Geometry: final body of the model. Coordinates: model frame, mm. A direction names the side the tool comes from. Give positions to 0.01 mm unless a question says otherwise; leave off trailing zeros. Write each loop counter-clockwise with the first axis right and the second up, starting at its lowest first coordinate (ties: lowest second). Pieces come first, ordered by that corner, then holes. Notation, with made-up numbers: (7.25, 63) -> (42.25, 63) arc R11 cw to (42.25, 83) -> close; hole circle Ø7 at (-7, -22). An arc over 180 degrees is marked (long way). Answer in a Markdown table with one row per item. Add a question column.
Item 1: Access query for faces 1 (the cylindrical face through (-88.645, 29.462, -31.871)), 2 (the cylindrical face through (-45.58, 1.04, -25.25)), 3 (the cylindrical face through (-84.923, 14.183, -34.226)). Directions: +Z, -Z, +X, -X, +Y, -Y. A direction counts if a zero-diameter tool reaches every point of the face in a straight line with its end or side. Return the directions, or none.
Item 2: Section query D-D on z = -28. State how many separate pieces and enclosed holes the cut face has, plus the area to 3 significant figures.
Item 3: First-contact query: P1, Ø1.5, axis at x = -87.5, z = -22, coming from the +Y side (3 decimals); P2, Ø1, axis at x = -77, z = -31, coming from the -Y side. Flat tips, straight axial feed; report the tip coordinate or a pass-through.
Item 4: Section query C-C on y = 20. Output: boundary loops of the cut face in (x, z).
Item 5: Section query A-A on y = 15.5. Output: boundary loops of the cut face in (x, z).
Item 6: Material intervals for probe 1 along X at (y, z) = (10, -29.75); probe 2 along Y at (x, z) = (-79, -20.25) (3 decimals); probe 3 along X at (y, z) = (16, -30.5), sorted ascending. Write a range as from..to.
Item 7: Draft query along X for faces 4 (the flat face through (-74, 19.05, -26)), 5 (the cylindrical face through (-64.645, 29.462, -31.871)), 6 (the flat face through (-44, 0, -27)). Return one class per face: +X half, -X half, draft (parallel to the pull), parting line (faces both ways), or undercut.
```python
from build123d import *

# Parameters (mm, degrees)
SKETCH1_W           = 55.5625
SKETCH1_H           = 31.75
BOSS_EXTRUDE1_DEPTH = 28.575
SKETCH2_R           = 7.62
CUT_EXTRUDE1_DEPTH  = 13.335
CUT_EXTRUDE2_DEPTH  = 12.7
SKETCH4_R           = 1.8415
CUT_EXTRUDE3_DEPTH  = 25.4
CUT_EXTRUDE4_DEPTH  = 17.78
SKETCH6_W           = 55.5625
SKETCH6_H           = 28.575
CUT_EXTRUDE5_DEPTH  = 15.875
SKETCH7_R           = 2.778125
CUT_EXTRUDE7_DEPTH  = 7.9375
SKETCH8_R           = 2.35
BOSS_EXTRUDE2_DEPTH = 1.8
SKETCH9_R           = 3.25
SKETCH9_R_2         = 2.425
CUT_EXTRUDE8_DEPTH  = 2.1


with BuildPart() as part:
    # Sketch1 → Boss-Extrude1 (new body)
    with BuildSketch(Plane(origin=(0, 0, 0), x_dir=(1, 0, 0), z_dir=(0, 1, 0))):
        with Locations((-66.667749699, 35.16562105)):
            Rectangle(SKETCH1_W, SKETCH1_H)
    extrude(amount=BOSS_EXTRUDE1_DEPTH)

    # Sketch2 → Cut-Extrude1 (cut)
    with BuildSketch(Plane.XY.offset(-19.29062105)):
        with Locations((-54.761499699, 14.2875)):
            Circle(SKETCH2_R)
    extrude(amount=-CUT_EXTRUDE1_DEPTH, mode=Mode.SUBTRACT)

    # Sketch3 → Cut-Extrude2 (cut)
    with BuildSketch(Plane.XY.offset(-19.29062105)):
        with BuildLine():
            Line((-80.161499699, 19.05), (-67.461499699, 19.05))
            ThreePointArc((-67.461499699, 19.05), (-62.698999699, 14.2875), (-67.461499699, 9.525))
            Line((-67.461499699, 9.525), (-80.161499699, 9.525))
            ThreePointArc((-80.161499699, 9.525), (-84.923999699, 14.2875), (-80.161499699, 19.05))
        make_face()
    extrude(amount=-CUT_EXTRUDE2_DEPTH, mode=Mode.SUBTRACT)

    # Sketch4 → Cut-Extrude3 (cut)
    with BuildSketch(Plane.XY.offset(-31.99062105)):
        with Locations((-80.161499699, 14.2875)):
            Circle(SKETCH4_R)
        with Locations((-67.461499699, 14.2875)):
            Circle(SKETCH4_R)
    extrude(amount=-CUT_EXTRUDE3_DEPTH, mode=Mode.SUBTRACT)

    # Sketch5 → Cut-Extrude4 (cut)
    with BuildSketch(Plane(origin=(0, 0, -51.04062105), x_dir=(-1, 0, 0), z_dir=(0, 0, -1))):
        with BuildLine():
            Line((67.461499699, 9.525), (80.161499699, 9.525))
            ThreePointArc((80.161499699, 9.525), (84.923999699, 14.2875), (80.161499699, 19.05))
            Line((80.161499699, 19.05), (67.461499699, 19.05))
            ThreePointArc((67.461499699, 19.05), (62.698999699, 14.2875), (67.461499699, 9.525))
        make_face()
    extrude(amount=-CUT_EXTRUDE4_DEPTH, mode=Mode.SUBTRACT)

    # Sketch6 → Cut-Extrude5 (cut)
    with BuildSketch(Plane(origin=(0, 0, -51.04062105), x_dir=(-1, 0, 0), z_dir=(0, 0, -1))):
        with Locations((66.667749699, 14.2875)):
            Rectangle(SKETCH6_W, SKETCH6_H)
    extrude(amount=-CUT_EXTRUDE5_DEPTH, mode=Mode.SUBTRACT)

    # Sketch7 → Cut-Extrude7 (cut)
    with BuildSketch(Plane.XY.offset(-32.62562105)):
        with Locations((-54.761499699, 14.2875)):
            Circle(SKETCH7_R)
    extrude(amount=-CUT_EXTRUDE7_DEPTH, mode=Mode.SUBTRACT)

    # Sketch8 → Boss-Extrude2 (add)
    with BuildSketch(Plane(origin=(0, 28.575, 0), x_dir=(1, 0, 0), z_dir=(0, 1, 0))):
        with Locations((-42.886499699, 31.16562105)):
            Circle(SKETCH8_R)
        with Locations((-42.886499699, 23.16562105)):
            Circle(SKETCH8_R)
        with Locations((-50.886499699, 31.16562105)):
            Circle(SKETCH8_R)
        with Locations((-50.886499699, 23.16562105)):
            Circle(SKETCH8_R)
        with Locations((-58.886499699, 31.16562105)):
            Circle(SKETCH8_R)
        with Locations((-58.886499699, 23.16562105)):
            Circle(SKETCH8_R)
        with Locations((-66.886499699, 31.16562105)):
            Circle(SKETCH8_R)
        with Locations((-66.886499699, 23.16562105)):
            Circle(SKETCH8_R)
        with Locations((-74.886499699, 31.16562105)):
            Circle(SKETCH8_R)
        with Locations((-74.886499699, 23.16562105)):
            Circle(SKETCH8_R)
        with Locations((-82.886499699, 31.16562105)):
            Circle(SKETCH8_R)
        with Locations((-82.886499699, 23.16562105)):
            Circle(SKETCH8_R)
        with Locations((-90.886499699, 31.16562105)):
            Circle(SKETCH8_R)
        with Locations((-90.886499699, 23.16562105)):
            Circle(SKETCH8_R)
    extrude(amount=BOSS_EXTRUDE2_DEPTH)

    # Sketch9 → Cut-Extrude8 (cut)
    with BuildSketch(Plane.XZ):
        Polygon((-82.874999699, -20.79062105), (-82.874999699, -20.49062105), (-90.148999699, -20.49062105), (-90.148999699, -20.79062105), (-90.748999699, -20.79062105), (-90.748999699, -20.49062105), (-93.248999699, -20.49062105), (-93.248999699, -22.99062105), (-92.948999699, -22.99062105), (-92.948999699, -23.59062105), (-93.248999699, -23.59062105), (-93.248999699, -30.99062105), (-92.948999699, -30.99062105), (-92.948999699, -31.59062105), (-93.248999699, -31.59062105), (-93.248999699, -33.96562105), (-90.748999699, -33.96562105), (-90.748999699, -33.66562105), (-90.148999699, -33.66562105), (-90.148999699, -33.96562105), (-82.874999699, -33.96562105), (-82.874999699, -33.66562105), (-82.274999699, -33.66562105), (-82.274999699, -33.96562105), (-75.000999699, -33.96562105), (-75.000999699, -33.66562105), (-74.400999699, -33.66562105), (-74.400999699, -33.96562105), (-67.126999699, -33.96562105), (-67.126999699, -33.66562105), (-66.526999699, -33.66562105), (-66.526999699, -33.96562105), (-59.252999699, -33.96562105), (-59.252999699, -33.66562105), (-58.652999699, -33.66562105), (-58.652999699, -33.96562105), (-51.378999699, -33.96562105), (-51.378999699, -33.66562105), (-50.778999699, -33.66562105), (-50.778999699, -33.96562105), (-43.504999699, -33.96562105), (-43.504999699, -33.66562105), (-42.904999699, -33.66562105), (-42.904999699, -33.96562105), (-40.086499699, -33.96562105), (-40.086499699, -20.49062105), (-42.904999699, -20.49062105), (-42.904999699, -20.79062105), (-43.504999699, -20.79062105), (-43.504999699, -20.49062105), (-50.778999699, -20.49062105), (-50.778999699, -20.79062105), (-51.378999699, -20.79062105), (-51.378999699, -20.49062105), (-58.652999699, -20.49062105), (-58.652999699, -20.79062105), (-59.252999699, -20.79062105), (-59.252999699, -20.49062105), (-66.526999699, -20.49062105), (-66.526999699, -20.79062105), (-67.126999699, -20.79062105), (-67.126999699, -20.49062105), (-74.400999699, -20.49062105), (-74.400999699, -20.79062105), (-75.000999699, -20.79062105), (-75.000999699, -20.49062105), (-82.274999699, -20.49062105), (-82.274999699, -20.79062105), align=None)
        with Locations((-86.886499699, -27.29062105)):
            Circle(SKETCH9_R, mode=Mode.SUBTRACT)
        with Locations((-78.886499699, -27.29062105)):
            Circle(SKETCH9_R, mode=Mode.SUBTRACT)
        with Locations((-70.886499699, -27.29062105)):
            Circle(SKETCH9_R, mode=Mode.SUBTRACT)
        with Locations((-62.886499699, -27.29062105)):
            Circle(SKETCH9_R, mode=Mode.SUBTRACT)
        with Locations((-54.886499699, -27.29062105)):
            Circle(SKETCH9_R, mode=Mode.SUBTRACT)
        with Locations((-46.886499699, -27.29062105)):
            Circle(SKETCH9_R, mode=Mode.SUBTRACT)
        with Locations((-46.886499699, -27.29062105)):
            Circle(SKETCH9_R_2)
        with Locations((-54.886499699, -27.29062105)):
            Circle(SKETCH9_R_2)
        with Locations((-62.886499699, -27.29062105)):
            Circle(SKETCH9_R_2)
        with Locations((-70.886499699, -27.29062105)):
            Circle(SKETCH9_R_2)
        with Locations((-78.886499699, -27.29062105)):
            Circle(SKETCH9_R_2)
        with Locations((-86.886499699, -27.29062105)):
            Circle(SKETCH9_R_2)
    extrude(amount=-CUT_EXTRUDE8_DEPTH, mode=Mode.SUBTRACT)


solid = part.part
```
Findings below:
| question | item | result |
|---|---|---|
| 1 | face 1 | +Y |
| 1 | face 2 | -Y |
| 1 | face 3 | -Z |
| 2 | separate pieces | 1 |
| 2 | enclosed holes | 2 |
| 2 | area | 1,120 mm^2 |
| 3 | P1 | stops at y = 28.575 |
| 3 | P2 | stops at y = 2.1 |
| 4 | outline | (-94.45, -35.17) -> (-38.89, -35.17) -> (-38.89, -19.29) -> (-49.72, -19.29) -> (-49.72, -32.63) -> (-59.8, -32.63) -> (-59.8, -19.29) -> (-94.45, -19.29) -> close |
| 5 | outline | (-94.45, -35.17) -> (-84.77, -35.17) -> (-84.77, -33.26) -> (-81.55, -33.26) -> (-81.55, -31.99) -> (-84.77, -31.99) -> (-84.77, -19.29) -> (-94.45, -19.29) -> close; (-78.78, -33.26) -> (-68.85, -33.26) -> (-68.85, -31.99) -> (-78.78, -31.99) -> close; (-66.08, -33.26) -> (-62.86, -33.26) -> (-62.86, -35.17) -> (-57.26, -35.17) -> (-57.26, -32.63) -> (-62.28, -32.63) -> (-62.28, -19.29) -> (-62.86, -19.29) -> (-62.86, -31.99) -> (-66.08, -31.99) -> close; (-52.26, -35.17) -> (-38.89, -35.17) -> (-38.89, -19.29) -> (-47.24, -19.29) -> (-47.24, -32.63) -> (-52.26, -32.63) -> close |
| 6 | probe 1 | x = -94.45..-82.23, -65.39..-61.06, -48.46..-38.89 |
| 6 | probe 2 | y = 0..9.525, 19.05..28.575 |
| 6 | probe 3 | x = -94.45..-84.61, -63.02..-62.19, -47.34..-38.89 |
| 7 | face 4 | undercut |
| 7 | face 5 | undercut |
| 7 | face 6 | draft |
